from build123d import *

# Parameters (mm, degrees)
SKETCH1_W           = 159
SKETCH1_H           = 118
BOSS_EXTRUDE1_DEPTH = 126
FILLET1_R           = 10
SKETCH6_W           = 80
SKETCH6_H           = 80
BOSS_EXTRUDE2_DEPTH = 30
SKETCH7_R           = 12
BOSS_EXTRUDE3_DEPTH = 40
SKETCH11_R          = 8.5
SKETCH11_R_2        = 10.5
CUT_EXTRUDE5_DEPTH  = 50
SKETCH12_R          = 7.94064545
CUT_EXTRUDE6_DEPTH  = 10


with BuildPart() as part:
    # Sketch1 → Boss-Extrude1 (new, symmetric)
    with BuildSketch(Plane.XY):
        Rectangle(SKETCH1_W, SKETCH1_H)
    extrude(amount=BOSS_EXTRUDE1_DEPTH, both=True)

    # Fillet1
    fillet1_edges = [part.edges().sort_by_distance(p)[0] for p in [
        (-79.5, 0, 126),
        (0, -59, 126),
        (79.5, 0, 126),
        (0, -59, -126),
        (-79.5, 0, -126),
        (0, 59, -126),
        (79.5, 0, -126),
        (0, 59, 126),
        (79.5, -59, 0),
        (-79.5, -59, 0),
        (-79.5, 59, 0),
        (79.5, 59, 0),
    ]]
    fillet(fillet1_edges, radius=FILLET1_R)

    # Sketch6 → Boss-Extrude2 (add)
    with BuildSketch(Plane(origin=(79.5, 0, 0), x_dir=(0, 0, -1), z_dir=(1, 0, 0))):
        with Locations((46.5, 0)):
            Rectangle(SKETCH6_W, SKETCH6_H)
    extrude(amount=BOSS_EXTRUDE2_DEPTH)

    # Sketch7 → Boss-Extrude3 (add)
    with BuildSketch(Plane(origin=(109.5, 0, 0), x_dir=(0, 0, -1), z_dir=(1, 0, 0))):
        with Locations((46.238380337, 0)):
            Circle(SKETCH7_R)
    extrude(amount=BOSS_EXTRUDE3_DEPTH)

    # Sketch11 → Cut-Extrude5 (cut)
    with BuildSketch(Plane.ZY.offset(79.5)):
        with Locations((93.08230214, 26.75)):
            Circle(SKETCH11_R)
        with Locations((93.08230214, -26.75)):
            Circle(SKETCH11_R_2)
    extrude(amount=-CUT_EXTRUDE5_DEPTH, mode=Mode.SUBTRACT)

    # Sketch12 → Cut-Extrude6 (cut)
    with BuildSketch(Plane.XZ.offset(59)):
        with Locations(Location((-38.5, -84, 0), (0, 0, 270))):
            Circle(SKETCH12_R)
        with Locations(Location((56.5, -84, 0), (0, 0, 270))):
            Circle(SKETCH12_R)
        with Locations(Location((56.5, -9, 0), (0, 0, 270))):
            Circle(SKETCH12_R)
        with Locations(Location((-38.5, -9, 0), (0, 0, 270))):
            Circle(SKETCH12_R)
    extrude(amount=-CUT_EXTRUDE6_DEPTH, mode=Mode.SUBTRACT)


solid = part.part
Here's how the part is built. I have some questions about the finished solid (model axes, mm). A direction names the side the tool comes from. Coordinates: 2 decimals unless noted, no trailing zeros. Order: outer loops, then holes, each group sorted by start corner. A loop starts at its lowest first (then second) coordinate and runs counter-clockwise, first axis right, second up. Notation, with made-up numbers: M 33.5,-11 L 45.5,-11 A21 cw 45.5,7 Z; hole C -40,49.5 d10. An arc over 180 degrees is marked long. Answer as CSV lines item,"result". Start each with the question number.
1. On a 3-axis mill with a long thin cutter (end or side, diameter ignored), from which of +Z, -Z, +X, -X, +Y, -Y can I reach the whole of each face in a straight line? I mean faces 4 (the flat face through (-38, -49, -84)), 5 (the flat face through (-29.5, -27, 93)), 6 (the flat face through (94, -40, -46)), 7 (the flat face through (94, 40, -46)). Say none if no direction works.
2. I want a section at D-D, the plane x = 84.5. Write out the boundary of the cut face in (y, z).
3. I need wall thicknesses on line 1 (Y direction, x = -38.5, z = 100); line 2 (X direction, y = -57, z = -9); line 3 (X direction, y = -56.75, z = -84). Which ranges of each line are inside material? Lowest first, please. Write a range as [from, to].
4. I want a section at A-A, the plane x = -38.5. Write out the boundary of the cut face in (y, z).
5. We'd pull the mould along X, two halves only. Please class faces 1 (the flat face through (109.5, 9, -37)), 2 (the cylindrical face through (-31.804, -54.07, -13.269)), 3 (the flat face through (-1, 59, 2)): released by +X, released by -X, zero draft, split by the parting line, or undercut.
6. For pin 1 (5 mm diameter, centred on y = 28, z = 90, fed in from -X); pin 2 (5 mm diameter, centred on x = 57.5, z = -11.5, fed in from -Y); pin 3 (5 mm diameter, centred on y = -2, z = 57.5, fed in from +X), each with a flat end and sliding along its axis, tell me the tip position at first contact or that it passes through.
7. I want a section at B-B, the plane y = 45. Write out the boundary of the cut face in (x, z).
8. I want a section at C-C, the plane z = 6. Write out the boundary of the cut face in (x, y).
Recorded:
1,face 4,"-Y"
1,face 5,"-X"
1,face 6,"+Z, -Z, +X, -Y"
1,face 7,"+Z, -Z, +X, +Y"
2,outline,"M -40,-86.5 L 40,-86.5 L 40,-6.5 L -40,-6.5 Z"
3,line 1,"y = [-59, -34.65], [-18.85, 21.81], [31.69, 59]"
3,line 2,"x = [-75.5, -46.44], [-30.56, 48.56], [64.44, 75.5]"
3,line 3,"x = [-75.82, -46.44], [-30.56, 48.56], [64.44, 75.82]"
4,outline,"M -59,-116 A10 ccw -49,-126 L 49,-126 A10 ccw 59,-116 L 59,116 A10 ccw 49,126 L -49,126 A10 ccw -59,116 L -59,-1.06 L -49,-1.06 L -49,-16.94 L -59,-16.94 L -59,-76.06 L -49,-76.06 L -49,-91.94 L -59,-91.94 Z; hole C -26.75,93.08 d21; hole C 26.75,93.08 d17"
5,face 1,"released by +X"
5,face 2,"undercut"
5,face 3,"zero draft"
6,pin 1,"stops at x = -29.5"
6,pin 2,"stops at y = -49"
6,pin 3,"stops at x = 79.5"
7,outline,"M -79.5,-116 A10 ccw -69.5,-126 L 69.5,-126 A10 ccw 79.5,-116 L 79.5,116 A10 ccw 69.5,126 L -69.5,126 A10 ccw -79.5,116 Z"
8,outline,"M -79.5,-49 A10 ccw -69.5,-59 L 69.5,-59 A10 ccw 79.5,-49 L 79.5,49 A10 ccw 69.5,59 L -69.5,59 A10 ccw -79.5,49 Z"
